Source: CAD feature listing. Evaluate the final solid. Frame: model axes, mm. Face numbers are marked on the shaded views. A direction names the side the tool comes from. Give positions to 0.01 mm unless a question says otherwise; leave off trailing zeros. Loops run counter-clockwise (first coordinate to the right, second up) from the corner with the lowest first, then second, coordinate; pieces in that order, holes last. Notation, with made-up numbers: M -39,78 L -27,78 A16 ccw -27,92 Z; hole C 34,40.25 d11. An arc over 180 degrees is marked long. Write item = value, one per line.
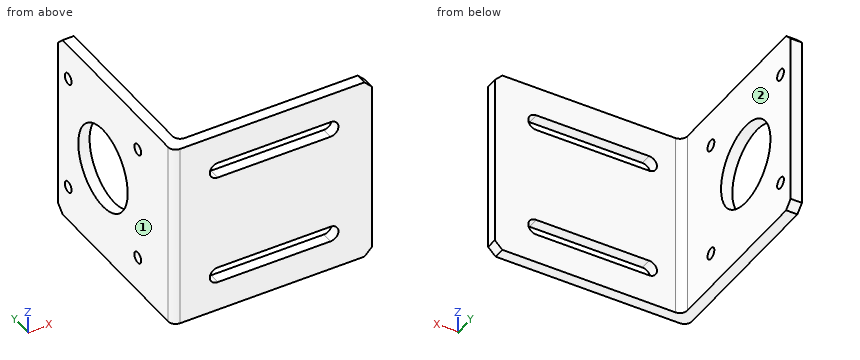
from build123d import *

# Parameters (mm, degrees)
Y_KSEKLIK_EKSTR_ZYON1_DEPTH = 50
IZIM2_R                     = 11
IZIM2_R_2                   = 1.5
KES_EKSTR_ZYON1_DEPTH       = 88.183714076
KES_EKSTR_ZYON2_DEPTH       = 88.252507127
KES_EKSTR_ZYON2_DEPTH_BACK  = 10
KES_EKSTR_ZYON3_DEPTH       = 88.183714076
KES_EKSTR_ZYON4_DEPTH       = 88.252507127


with BuildPart() as part:
    # Çizim1 → Yükseklik-Ekstrüzyon1 (new body)
    with BuildSketch(Plane.XY):
        with BuildLine():
            Line((0, 51), (0, 2))
            ThreePointArc((0, 2), (0.585786438, 0.585786438), (2, 0))
            Line((2, 0), (53, 0))
            Line((53, 0), (53, 3))
            Line((53, 3), (5, 3))
            ThreePointArc((5, 3), (3.585786438, 3.585786438), (3, 5))
            Line((3, 5), (3, 51))
            Line((3, 51), (0, 51))
        make_face()
    extrude(amount=Y_KSEKLIK_EKSTR_ZYON1_DEPTH)

    # Çizim2 → Kes-Ekstrüzyon1 (cut, through all)
    with BuildSketch(Plane(origin=(3, 0, 0), x_dir=(0, 0, -1), z_dir=(1, 0, 0))):
        with Locations((-25, 31)):
            Circle(IZIM2_R)
        with Locations((-9.5, 46.5)):
            Circle(IZIM2_R_2)
        with Locations(Location((-40.5, 46.5, 0), (0, 0, 180))):
            Circle(IZIM2_R_2)
        with Locations(Location((-9.5, 15.5, 0), (0, 0, 180))):
            Circle(IZIM2_R_2)
        with Locations((-40.5, 15.5)):
            Circle(IZIM2_R_2)
    extrude(amount=-KES_EKSTR_ZYON1_DEPTH, mode=Mode.SUBTRACT)

    # Çizim3 → Kes-Ekstrüzyon2 (cut, two sides: drawn at the far end of the back side and taken through both)
    with BuildSketch(Plane(origin=(0, 3, 0), x_dir=(1, 0, 0), z_dir=(0, 1, 0)).offset(-KES_EKSTR_ZYON2_DEPTH_BACK)):
        with BuildLine():
            Line((42, -12.1), (12, -12.1))
            ThreePointArc((12, -12.1), (9.9, -10), (12, -7.9))
            Line((12, -7.9), (42, -7.9))
            ThreePointArc((42, -7.9), (44.1, -10), (42, -12.1))
        make_face()
        with BuildLine():
            Line((42, -37.9), (12, -37.9))
            ThreePointArc((12, -37.9), (9.9, -40), (12, -42.1))
            Line((12, -42.1), (42, -42.1))
            ThreePointArc((42, -42.1), (44.1, -40), (42, -37.9))
        make_face()
    extrude(amount=KES_EKSTR_ZYON2_DEPTH + KES_EKSTR_ZYON2_DEPTH_BACK, mode=Mode.SUBTRACT)

    # Çizim4 → Kes-Ekstrüzyon3 (cut, through all)
    with BuildSketch(Plane(origin=(3, 0, 0), x_dir=(0, 0, -1), z_dir=(1, 0, 0))):
        Polygon((-50, 49), (-50, 51), (-48, 51), align=None)
        Polygon((0, 49), (0, 51), (-2, 51), align=None)
    extrude(amount=-KES_EKSTR_ZYON3_DEPTH, mode=Mode.SUBTRACT)

    # Çizim5 → Kes-Ekstrüzyon4 (cut, through all)
    with BuildSketch(Plane(origin=(0, 3, 0), x_dir=(1, 0, 0), z_dir=(0, 1, 0))):
        Polygon((53, -48), (51, -50), (53, -50), align=None)
        Polygon((53, 0), (53, -2), (51, 0), align=None)
    extrude(amount=-KES_EKSTR_ZYON4_DEPTH, mode=Mode.SUBTRACT)


solid = part.part
1. Cut plane D-D, the plane y = 46.5. Return the cut outline in (x, z), then the cut area to 3 significant figures.
Derived:
outline = M 0,0 L 3,0 L 3,8 L 0,8 Z; M 0,11 L 3,11 L 3,39 L 0,39 Z; M 0,42 L 3,42 L 3,50 L 0,50 Z
area = 132 mm²
2. Material intervals for probe 1 along Y at (x, z) = (1.3, 9.5); probe 2 along Y at (x, z) = (1, 40); probe 3 along X at (y, z) = (38, 15), sorted ascending. Write a range as from..to.
Derived:
probe_1 = 0.13..14, 17..45, 48..51
probe_2 = 0.27..14.09, 16.91..45.09, 47.91..51
probe_3 = 0..3
3. Cut plane C-C, the plane x = 24.5. Return the cut outline in (y, z), then the cut area to 3 significant figures.
Derived:
outline = M 0,0 L 3,0 L 3,7.9 L 0,7.9 Z; M 0,12.1 L 3,12.1 L 3,37.9 L 0,37.9 Z; M 0,42.1 L 3,42.1 L 3,50 L 0,50 Z
area = 125 mm²
4. Cut plane B-B, the plane z = 25. Return the cut outline in (x, y), then the cut area to 3 significant figures.
Derived:
outline = M 0,2 A2 ccw 2,0 L 53,0 L 53,3 L 5,3 A2 cw 3,5 L 3,20 L 0,20 Z; M 0,42 L 3,42 L 3,51 L 0,51 Z
area = 237 mm²
5. Reachability of the marked faces 1 and 2 from +Z, -Z, +X, -X, +Y, -Y: full face, straight path, thin tool, end or side. Return the list, or none.
Derived:
face_1 = +Z, -Z, -X, +Y, -Y
face_2 = +Z, -Z, +X, +Y
6. Cut plane A-A, the plane y = 31. Return the cut outline in (x, z).
Derived:
outline = M 0,0 L 3,0 L 3,14 L 0,14 Z; M 0,36 L 3,36 L 3,50 L 0,50 Z
7. First-contact query: pin 1 Ø3.5 at (y, z) = (15.5, 9.5) entering from +X; pin 2 Ø2.5 at (y, z) = (46.5, 40.5) entering from -X; pin 3 Ø1 at (x, z) = (37, 30) entering from +Y. Flat tips, straight axial feed; report the tip coordinate or a pass-through.
Derived:
pin_1 = 3
pin_2 = through
pin_3 = 3
